from build123d import *

# Parameters (mm, degrees)
SKETCH1_R             = 14
SKETCH1_R_2           = 10
BOSS_EXTRUDE2_DEPTH   = 3
BOSS_EXTRUDE2_2_DEPTH = 3
BOSS_EXTRUDE2_3_DEPTH = 3
BOSS_EXTRUDE2_4_DEPTH = 3
SKETCH2_W             = 100
SKETCH2_H             = 65
BOSS_EXTRUDE3_DEPTH   = 15
BOSS_EXTRUDE4_DEPTH   = 20
SKETCH4_R             = 20
BOSS_EXTRUDE5_DEPTH   = 5.5
BOSS_EXTRUDE6_START   = -23
SKETCH5_R             = 20
BOSS_EXTRUDE6_DEPTH   = 23
SKETCH6_R             = 15
BOSS_EXTRUDE7_DEPTH   = 5
SKETCH7_R             = 10
CUT_EXTRUDE1_DEPTH    = 120.825265291
BOSS_EXTRUDE8_DEPTH   = 6.5
SKETCH13_R            = 10
CUT_EXTRUDE2_DEPTH    = 113.463746168


with BuildPart() as part:
    # Sketch1 → Boss-Extrude2 (new body)
    with BuildSketch(Plane(origin=(0, 0, 0), x_dir=(1, 0, 0), z_dir=(0, 1, 0))):
        with Locations(Location((50.63816244, 20.825493171, 0), (0, 0, 270))):
            Circle(SKETCH1_R)
        with Locations(Location((50.63816244, 20.825493171, 0), (0, 0, 270))):
            Circle(SKETCH1_R_2, mode=Mode.SUBTRACT)
    extrude(amount=BOSS_EXTRUDE2_DEPTH)



with BuildPart() as body_2:
    # Sketch1 → Boss-Extrude2 2 (new body)
    with BuildSketch(Plane(origin=(0, 0, 0), x_dir=(1, 0, 0), z_dir=(0, 1, 0))):
        with Locations(Location((50.63816244, -16.174506829, 0), (0, 0, 270))):
            Circle(SKETCH1_R)
        with Locations(Location((50.63816244, -16.174506829, 0), (0, 0, 270))):
            Circle(SKETCH1_R_2, mode=Mode.SUBTRACT)
    extrude(amount=BOSS_EXTRUDE2_2_DEPTH)


with BuildPart() as body_3:
    # Sketch1 → Boss-Extrude2 3 (new body)
    with BuildSketch(Plane(origin=(0, 0, 0), x_dir=(1, 0, 0), z_dir=(0, 1, 0))):
        with Locations(Location((-21.36183756, 20.825493171, 0), (0, 0, 270))):
            Circle(SKETCH1_R)
        with Locations(Location((-21.36183756, 20.825493171, 0), (0, 0, 270))):
            Circle(SKETCH1_R_2, mode=Mode.SUBTRACT)
    extrude(amount=BOSS_EXTRUDE2_3_DEPTH)


with BuildPart() as body_4:
    # Sketch1 → Boss-Extrude2 4 (new body)
    with BuildSketch(Plane(origin=(0, 0, 0), x_dir=(1, 0, 0), z_dir=(0, 1, 0))):
        with Locations(Location((-21.36183756, -16.174506829, 0), (0, 0, 270))):
            Circle(SKETCH1_R)
        with Locations(Location((-21.36183756, -16.174506829, 0), (0, 0, 270))):
            Circle(SKETCH1_R_2, mode=Mode.SUBTRACT)
    extrude(amount=BOSS_EXTRUDE2_4_DEPTH)


with BuildPart() as part_1:
    add(part.part)

    add(body_2.part)  # Boss-Extrude3 merges body 2

    add(body_3.part)  # Boss-Extrude3 merges body 3

    add(body_4.part)  # Boss-Extrude3 merges body 4
    # Sketch2 → Boss-Extrude3 (add)
    with BuildSketch(Plane(origin=(0, 0, 0), x_dir=(1, 0, 0), z_dir=(0, 1, 0))):
        with Locations((14.63816244, 2.325493171)):
            Rectangle(SKETCH2_W, SKETCH2_H)
    extrude(amount=-BOSS_EXTRUDE3_DEPTH)

    # Sketch3 → Boss-Extrude4 (add, symmetric)
    with BuildSketch(Plane(origin=(14.63816244, 0, 0), x_dir=(0, 0, -1), z_dir=(1, 0, 0))):
        with BuildLine():
            Line((-30.174506829, 12), (-30.174506829, 0))
            Line((-30.174506829, 0), (-18.174506829, 0))
            Line((-18.174506829, 0), (-18.174506829, 10.52211824))
            ThreePointArc((-18.174506829, 10.52211824), (-26.203196706, 30.629306034), (-46.170428478, 39))
            Line((-46.170428478, 39), (-57.587061699, 39))
            Line((-57.587061699, 39), (-57.587061699, 27))
            Line((-57.587061699, 27), (-45.174506829, 27))
            ThreePointArc((-45.174506829, 27), (-34.567905111, 22.606601718), (-30.174506829, 12))
        make_face()
    extrude(amount=BOSS_EXTRUDE4_DEPTH, both=True)

    # Sketch4 → Boss-Extrude5 (add)
    with BuildSketch(Plane(origin=(0, 39, 0), x_dir=(1, 0, 0), z_dir=(0, 1, 0))):
        with Locations(Location((14.63816244, -57.587061699, 0), (0, 0, 145.191759612))):
            Circle(SKETCH4_R)
    extrude(amount=BOSS_EXTRUDE5_DEPTH)

    # Sketch5 → Boss-Extrude6 (add)
    with BuildSketch(Plane(origin=(0, 44.5, 0), x_dir=(1, 0, 0), z_dir=(0, 1, 0)).offset(BOSS_EXTRUDE6_START)):
        with Locations(Location((14.63816244, -57.587061699, 0), (0, 0, 270))):
            Circle(SKETCH5_R)
    extrude(amount=BOSS_EXTRUDE6_DEPTH)

    # Sketch6 → Boss-Extrude7 (add)
    with BuildSketch(Plane(origin=(0, 44.5, 0), x_dir=(1, 0, 0), z_dir=(0, 1, 0))):
        with Locations(Location((14.63816244, -57.587061699, 0), (0, 0, 270))):
            Circle(SKETCH6_R)
    extrude(amount=BOSS_EXTRUDE7_DEPTH)

    # Sketch7 → Cut-Extrude1 (cut, through all)
    with BuildSketch(Plane(origin=(0, 49.5, 0), x_dir=(1, 0, 0), z_dir=(0, 1, 0))):
        with Locations(Location((14.63816244, -57.587061699, 0), (0, 0, 270))):
            Circle(SKETCH7_R)
    extrude(amount=-CUT_EXTRUDE1_DEPTH, mode=Mode.SUBTRACT)


with BuildPart() as boss_extrude8_tool:
    # Sketch12 → Boss-Extrude8 (new, symmetric)
    with BuildSketch(Plane(origin=(14.63816244, 0, 0), x_dir=(0, 0, -1), z_dir=(1, 0, 0))):
        with BuildLine():
            Line((-18.170428478, 11), (-18.174506829, 3))
            Line((-18.174506829, 3), (-18.174506829, 0))
            Line((-18.174506829, 0), (31.654695104, 0))
            Line((31.654695104, 0), (34.825493171, 0))
            ThreePointArc((34.825493171, 0), (4.909491405, 32.485841169), (-37.587061699, 44.5))
            Line((-37.587061699, 44.5), (-42.002826433, 44.5))
            Line((-42.002826433, 44.5), (-42.002826433, 38.688103821))
            ThreePointArc((-42.002826433, 38.688103821), (-39.774060831, 38.259017893), (-37.587061699, 37.651938292))
            ThreePointArc((-37.587061699, 37.651938292), (-23.535561338, 27.490091956), (-18.170428478, 11))
        make_face()
    extrude(amount=BOSS_EXTRUDE8_DEPTH, both=True)


with BuildPart() as part_2:
    add(part_1.part)


with BuildPart() as part_3:
    # Boss-Extrude8: joined with boss_extrude8_tool
    add(part_2.part.fuse(boss_extrude8_tool.part, tol=0.00001))

    # Sketch13 → Cut-Extrude2 (cut, through all)
    with BuildSketch(Plane(origin=(0, 0, 0), x_dir=(1, 0, 0), z_dir=(0, 1, 0))):
        with Locations(Location((-21.36183756, 20.825493171, 0), (0, 0, 270))):
            Circle(SKETCH13_R)
        with Locations(Location((-21.36183756, -16.174506829, 0), (0, 0, 270))):
            Circle(SKETCH13_R)
        with Locations(Location((50.63816244, 20.825493171, 0), (0, 0, 270))):
            Circle(SKETCH13_R)
        with Locations(Location((50.63816244, -16.174506829, 0), (0, 0, 270))):
            Circle(SKETCH13_R)
    extrude(amount=-CUT_EXTRUDE2_DEPTH, mode=Mode.SUBTRACT)


solid = part_3.part
Here's how the part is built. I have some questions about the finished solid (model axes, mm). A direction names the side the tool comes from. Coordinates: 2 decimals unless noted, no trailing zeros. Loops run counter-clockwise (first coordinate to the right, second up) from the corner with the lowest first, then second, coordinate; pieces in that order, holes last.
1. Imagine slicing it at C-C, the plane z = 9. Please give me the cut outline in (x, y).
2. For P1, Ø6, axis at y = 12, z = 6.5, coming from the +X side; P2, Ø12, axis at y = 29, z = 34, coming from the -X side; P3, Ø5, axis at x = 17, z = 36, coming from the -Y side, each with a flat end and sliding along its axis, tell me the tip position at first contact or that it passes through.
3. Imagine slicing it at B-B, the plane x = 56. Please give me the cut outline in (y, z), and give its area (3 significant figures).
4. For faces 1 (the cylindrical face through (64.52, 1.48, 14.35)), 2 (the flat face through (62, 0, 27)), 3 (the flat face through (-30, 3, 22)), 4 (the flat face through (33, 27, 48)), which set-ups out of +Z, -Z, +X, -X, +Y, -Y let a thin tool reach every point of the face, with its end or its side?
5. Imagine slicing it at D-D, the plane y = 25. Please give me the cut outline in (x, z).
6. Imagine slicing it at A-A, the plane y = -7.5. Please give me the cut outline in (x, z), and give its area (3 significant figures).
7. I need wall thicknesses on L1, parallel to X at y = -12, z = 12; L2, parallel to Y at x = 22.5, z = 4; L3, parallel to X at y = 29.5, z = 57. Which ranges of each line are inside material? Lowest first, please.
Taken from the geometry:
1. outline: (-35.36, -15) - (-28.33, -15) - (-28.33, 3) - (-33.38, 3) - (-33.38, 0) - (-35.36, 0) - close; (-14.4, -15) - (43.67, -15) - (43.67, 3) - (38.62, 3) - (38.62, 0) - (21.14, 0) - (21.14, 39.3) - (8.14, 39.3) - (8.14, 0) - (-9.34, 0) - (-9.34, 3) - (-14.4, 3) - close; (57.6, -15) - (64.64, -15) - (64.64, 0) - (62.66, 0) - (62.66, 3) - (57.6, 3) - close
2. P1: stops at x = 21.14
2. P2: stops at x = -5.36
2. P3: stops at y = 21.42
3. outline: (-15, -34.83) - (0, -34.83) - (0, -33.76) - (3, -33.76) - (3, -29.27) - (-15, -29.27) - close; (-15, -12.38) - (3, -12.38) - (3, -7.89) - (0, -7.89) - (0, 3.24) - (3, 3.24) - (3, 7.73) - (-15, 7.73) - close; (-15, 24.62) - (3, 24.62) - (3, 29.11) - (0, 29.11) - (0, 30.17) - (-15, 30.17) - close
3. area: 522 mm2
4. face 1: +Y
4. face 2: +Z, +X, +Y
4. face 3: +Z, -Z, -X, +Y
4. face 4: +X, -Y
5. outline: (-5.36, 21.92) - (34.64, 21.92) - (34.64, 37.69) - (16.68, 37.69) arc R20 ccw (long way) to (12.6, 37.69) - (-5.36, 37.69) - close; (8.14, -15.19) - (21.14, -15.19) - (21.14, 21.92) - (8.14, 21.92) - close; hole circle Ø20 at (14.64, 57.59)
6. outline: (-35.36, -34.83) - (64.64, -34.83) - (64.64, 30.17) - (-35.36, 30.17) - close; hole circle Ø20 at (-21.36, -20.83); hole circle Ø20 at (-21.36, 16.17); hole circle Ø20 at (50.64, -20.83); hole circle Ø20 at (50.64, 16.17)
6. area: 5,240 mm2
7. L1: x = -35.36 to -30.45, -12.27 to 41.55, 59.73 to 64.64
7. L2: y = -15 to 0
7. L3: x = -5.36 to 4.66, 24.62 to 34.64
